Could you check a few things on this model? Use its own coordinates, in mm. Face numbers are marked on the shaded views. Coordinates: 2 decimals unless noted, no trailing zeros. Order: outer loops, then holes, each group sorted by start corner. A loop starts at its lowest first (then second) coordinate and runs counter-clockwise, first axis right, second up. Notation, with made-up numbers: (40, 53) - (59, 53) arc R8 cw to (59, 63) - close; hole circle Ø2 at (84, -22). An arc over 180 degrees is marked (long way). Answer as CSV lines item,"result". Start each with the question number.
1. Thinking about a two-plate mould opening in Y: for the marked faces 1 and 2, which applies, released by +Y, released by -Y, zero draft, split by the parting line, or undercut?
2. I want a section at B-B, the plane x = 109. List the corners of the cut face in (y, z) for me, and give its area (3 significant figures).
3. I want a section at C-C, the plane y = 48.5. List the corners of the cut face in (x, z) for me, and give its area (3 significant figures).
4. I need wall thicknesses on probe 1 along X at (y, z) = (27, -1); probe 2 along Y at (x, z) = (125.5, -0.9); probe 3 along Y at (x, z) = (-107.5, -7.5). Which ranges of each line are inside material? Lowest first, please.
5. I want a section at A-A, the plane y = 79. List the corners of the cut face in (x, z) for me, and give its area (3 significant figures).
6. For pin 1 (8 mm diameter, centred on x = 105, y = 23, fed in from +Z); pin 2 (4.5 mm diameter, centred on x = -124.5, z = -7.24, fed in from +Y); pin 3 (2 mm diameter, centred on x = 12.5, z = -1, fed in from -Y); pin 4 (1.6 mm diameter, centred on x = 22, z = -1.5, fed in from +Y), each with a flat end and sliding along its axis, tell me the tip position at first contact or that it passes through.
from build123d import *

# Parameters (mm, degrees)
SKETCH2_W                      = 309
SKETCH2_H                      = 106
BASE_FLANGE1_DEPTH             = 2
EDGE_FLANGE1_STRIP_W           = 9.4732
EDGE_FLANGE1_STRIP_H           = 2
EDGE_FLANGE1_STRIP_CUT_DEPTH   = 309
EDGE_FLANGE1_STRIP_2_W         = 9.4732
EDGE_FLANGE1_STRIP_2_H         = 2
EDGE_FLANGE1_STRIP_CUT_2_DEPTH = 309
EDGE_FLANGE1_DEPTH             = 309
EDGE_FLANGE1_BEND_DEPTH        = 309
CUT_EXTRUDE1_DEPTH             = 188.750499334
CUT_EXTRUDE1_DEPTH_BACK        = 188.750499334
SKETCH13_R                     = 12
CUT_EXTRUDE2_DEPTH             = 188.750499334
CUT_EXTRUDE2_DEPTH_BACK        = 188.750499334
SKETCH14_W                     = 78.027092835
SKETCH14_H                     = 15
CUT_EXTRUDE3_DEPTH             = 188.750499334
CUT_EXTRUDE3_DEPTH_BACK        = 188.750499334
SKETCH15_R                     = 2.5


# Sheet-metal steps are written as plain solids
with BuildPart() as part:
    # Sketch2 → Base-Flange1 (new body)
    with BuildSketch(Plane.XY):
        with Locations((0, 53)):
            Rectangle(SKETCH2_W, SKETCH2_H)
    extrude(amount=-BASE_FLANGE1_DEPTH)

    # Edge-Flange1 strip (across the edge) → Edge-Flange1 strip cut (cut)
    with BuildSketch(Plane(origin=(154.5, 0, -2), x_dir=(0, 1, 0), z_dir=(-1, 0, 0))):
        with Locations((-2, -1)):
            Rectangle(EDGE_FLANGE1_STRIP_W, EDGE_FLANGE1_STRIP_H)
    extrude(amount=EDGE_FLANGE1_STRIP_CUT_DEPTH, mode=Mode.SUBTRACT)

    # Edge-Flange1 strip 2 (across the edge) → Edge-Flange1 strip cut 2 (cut)
    with BuildSketch(Plane(origin=(-154.5, 106, -2), x_dir=(0, -1, 0), z_dir=(1, 0, 0))):
        with Locations((-2, -1)):
            Rectangle(EDGE_FLANGE1_STRIP_2_W, EDGE_FLANGE1_STRIP_2_H)
    extrude(amount=EDGE_FLANGE1_STRIP_CUT_2_DEPTH, mode=Mode.SUBTRACT)

    # Edge-Flange1 section (across the edge) → Edge-Flange1 (add)
    with BuildSketch(Plane(origin=(154.5, 0, -2), x_dir=(0, 1, 0), z_dir=(-1, 0, 0))):
        with BuildLine():
            Line((0, 0.7366), (0, 10))
            Line((0, 10), (2, 10))
            Line((2, 10), (2, 0.7366))
            ThreePointArc((2, 0.7366), (2.215745145, 0.215745145), (2.7366, 0))
            Line((2.7366, 0), (2.7366, -2))
            ThreePointArc((2.7366, -2), (0.801531583, -1.198468417), (0, 0.7366))
        make_face()
    extrude(amount=EDGE_FLANGE1_DEPTH)

    # Edge-Flange1 section 2 (across the edge) → Edge-Flange1 bend (add)
    with BuildSketch(Plane(origin=(-154.5, 106, -2), x_dir=(0, -1, 0), z_dir=(1, 0, 0))):
        with BuildLine():
            Line((0, 0.7366), (0, 10))
            Line((0, 10), (2, 10))
            Line((2, 10), (2, 0.7366))
            ThreePointArc((2, 0.7366), (2.215745145, 0.215745145), (2.7366, 0))
            Line((2.7366, 0), (2.7366, -2))
            ThreePointArc((2.7366, -2), (0.801531583, -1.198468417), (0, 0.7366))
        make_face()
    extrude(amount=EDGE_FLANGE1_BEND_DEPTH)

    # Sketch13 → Cut-Extrude1 (cut, two sides: drawn at the far end of the back side and taken through both)
    with BuildSketch(Plane.XY.offset(-CUT_EXTRUDE1_DEPTH_BACK)):
        with Locations((125.5, 79)):
            Circle(SKETCH13_R)
        with Locations((125.5, 27)):
            Circle(SKETCH13_R)
    extrude(amount=CUT_EXTRUDE1_DEPTH + CUT_EXTRUDE1_DEPTH_BACK, mode=Mode.SUBTRACT)

    # Sketch14 → Cut-Extrude2 (cut, two sides: drawn at the far end of the back side and taken through both)
    with BuildSketch(Plane.XY.offset(-CUT_EXTRUDE2_DEPTH_BACK)):
        with Locations((30.773130234, 90.5)):
            Rectangle(SKETCH14_W, SKETCH14_H)
    extrude(amount=CUT_EXTRUDE2_DEPTH + CUT_EXTRUDE2_DEPTH_BACK, mode=Mode.SUBTRACT)

    # Sketch15 → Cut-Extrude3 (cut, two sides: drawn at the far end of the back side and taken through both)
    with BuildSketch(Plane(origin=(0, 106, 0), x_dir=(1, 0, 0), z_dir=(0, 1, 0)).offset(-CUT_EXTRUDE3_DEPTH_BACK)):
        with Locations(Location((124.5, 7.2366, 0), (0, 0, 90))):
            Circle(SKETCH15_R)
        with Locations(Location((0, 7.2366, 0), (0, 0, 90))):
            Circle(SKETCH15_R)
        with Locations(Location((-124.5, 7.2366, 0), (0, 0, 90))):
            Circle(SKETCH15_R)
    extrude(amount=CUT_EXTRUDE3_DEPTH + CUT_EXTRUDE3_DEPTH_BACK, mode=Mode.SUBTRACT)


solid = part.part
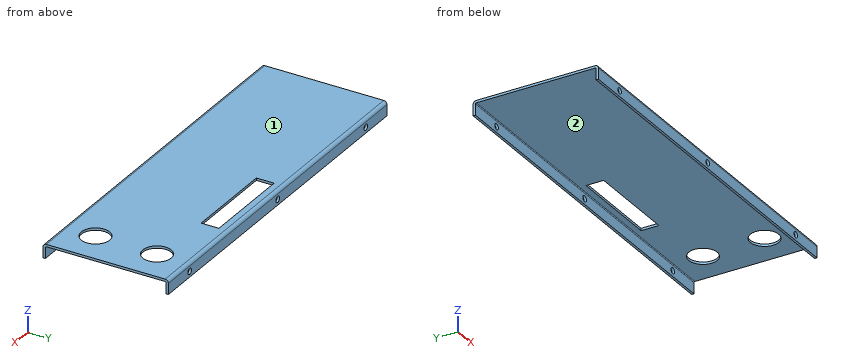
Solved:
1,face 1,"zero draft"
1,face 2,"undercut"
2,outline,"(0, -12) - (2, -12) - (2, -2.74) arc R0.74 cw to (2.74, -2) - (103.26, -2) arc R0.74 cw to (104, -2.74) - (104, -12) - (106, -12) - (106, -2.74) arc R2.74 ccw to (103.26, 0) - (2.74, 0) arc R2.74 ccw to (0, -2.74) - close"
2,area,"249 mm2"
3,outline,"(-154.5, -2) - (154.5, -2) - (154.5, 0) - (-154.5, 0) - close"
3,area,"618 mm2"
4,probe 1,"x = -154.5 to 113.5, 137.5 to 154.5"
4,probe 2,"y = 0.71 to 15, 39 to 67, 91 to 105.29"
4,probe 3,"y = 0 to 2, 104 to 106"
5,outline,"(-154.5, -2) - (113.5, -2) - (113.5, 0) - (-154.5, 0) - close; (137.5, -2) - (154.5, -2) - (154.5, 0) - (137.5, 0) - close"
5,area,"570 mm2"
6,pin 1,"stops at z = 0"
6,pin 2,"passes through"
6,pin 3,"stops at y = 0.1"
6,pin 4,"stops at y = 105.96"
